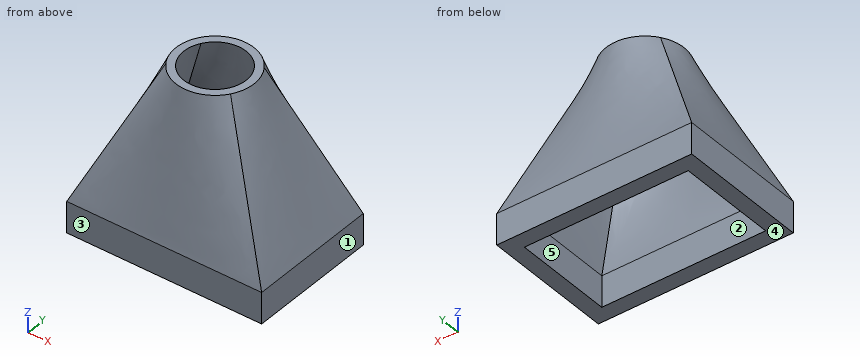
```python
from build123d import *

# Parameters (mm, degrees)
SKETCH1_W           = 12.5
SKETCH1_H           = 8.4
SKETCH1_W_2         = 10.5
SKETCH1_H_2         = 6.4
BOSS_EXTRUDE1_DEPTH = 1
SKETCH6_W           = 12.5
SKETCH6_H           = 8.4
BOSS_EXTRUDE2_DEPTH = 1
SKETCH7_W           = 10.5
SKETCH7_H           = 6.4
CUT_EXTRUDE1_DEPTH  = 1


with BuildPart() as part:
    # Sketch1 → Boss-Extrude1 (new body)
    with BuildSketch(Plane.XY):
        Rectangle(SKETCH1_W, SKETCH1_H)
        Rectangle(SKETCH1_W_2, SKETCH1_H_2, mode=Mode.SUBTRACT)
    extrude(amount=BOSS_EXTRUDE1_DEPTH)

    # Sketch3 → Loft1 section 0
    with BuildSketch(Plane.XY.offset(1)):
        with BuildLine():
            Line((6.25, -4.2), (6.25, 4.2))
            Line((6.25, 4.2), (-6.25, 4.2))
            Line((-6.25, 4.2), (-6.25, -4.2))
            Line((-6.25, -4.2), (6.25, -4.2))
        make_face()
    # Sketch2 for Loft1 → Loft1 section 1
    with BuildSketch(Plane.XY.offset(10)):
        with BuildLine():
            # circular arc as an exact rational Bezier (weights 1, cos(half-angle), 1)
            Bezier((2.075003924, -1.394402637), (3.012042497, 0), (2.075003924, 1.394402637), weights=[1, 0.830001569, 1])
            Bezier((2.075003924, 1.394402637), (0, 4.482206096), (-2.075003924, 1.394402637), weights=[1, 0.557761055, 1])
            Bezier((-2.075003924, 1.394402637), (-3.012042497, 0), (-2.075003924, -1.394402637), weights=[1, 0.830001569, 1])
            Bezier((-2.075003924, -1.394402637), (0, -4.482206096), (2.075003924, -1.394402637), weights=[1, 0.557761055, 1])
        make_face()
    loft()

    # Cut-Loft1: read off the stored shape, not the designer's step
    # Cut-Loft1: loft between two sections, ruled curve by curve
    cut_loft1_from = [
        Edge.make_bspline([(1.707768655, -1.040925656, 10), (1.633699479, -1.162445397, 10), (1.542008876, -1.28354475, 10), (1.31984949, -1.511051231, 10), (1.189256111, -1.617336715, 10), (0.892947872, -1.797985608, 10), (0.72722112, -1.87212471, 10), (0.374256765, -1.973229171, 10), (0.187198335, -2, 10), (-0.187198335, -2, 10), (-0.374256765, -1.973229171, 10), (-0.72722112, -1.87212471, 10), (-0.892947872, -1.797985608, 10), (-1.189256111, -1.617336715, 10), (-1.31984949, -1.511051231, 10), (-1.542008876, -1.28354475, 10), (-1.633699479, -1.162445397, 10), (-1.707768655, -1.040925656, 10)], [0, 0, 0, 0, 0.125, 0.125, 0.25, 0.25, 0.375, 0.375, 0.5, 0.5, 0.625, 0.625, 0.75, 0.75, 0.875, 0.875, 1, 1, 1, 1], 3),
        Edge.make_bspline([(-1.707768655, -1.040925656, 10), (-1.798062507, -0.892787306, 10), (-1.872174068, -0.727085204, 10), (-1.973239973, -0.374182636, 10), (-2, -0.187161202, 10), (-2, 0.187161202, 10), (-1.973239973, 0.374182636, 10), (-1.872174068, 0.727085204, 10), (-1.798062507, 0.892787306, 10), (-1.707768655, 1.040925656, 10)], [0, 0, 0, 0, 0.25, 0.25, 0.5, 0.5, 0.75, 0.75, 1, 1, 1, 1], 3),
        Edge.make_bspline([(1.707768655, 1.040925656, 10), (1.798062507, 0.892787306, 10), (1.872174068, 0.727085204, 10), (1.973239973, 0.374182636, 10), (2, 0.187161202, 10), (2, -0.187161202, 10), (1.973239973, -0.374182636, 10), (1.872174068, -0.727085204, 10), (1.798062507, -0.892787306, 10), (1.707768655, -1.040925656, 10)], [0, 0, 0, 0, 0.25, 0.25, 0.5, 0.5, 0.75, 0.75, 1, 1, 1, 1], 3),
        Edge.make_bspline([(-1.707768655, 1.040925656, 10), (-1.633699479, 1.162445397, 10), (-1.542008876, 1.28354475, 10), (-1.31984949, 1.511051231, 10), (-1.189256111, 1.617336715, 10), (-0.892947872, 1.797985608, 10), (-0.72722112, 1.87212471, 10), (-0.374256765, 1.973229171, 10), (-0.187198335, 2, 10), (0.187198335, 2, 10), (0.374256765, 1.973229171, 10), (0.72722112, 1.87212471, 10), (0.892947872, 1.797985608, 10), (1.189256111, 1.617336715, 10), (1.31984949, 1.511051231, 10), (1.542008876, 1.28354475, 10), (1.633699479, 1.162445397, 10), (1.707768655, 1.040925656, 10)], [0, 0, 0, 0, 0.125, 0.125, 0.25, 0.25, 0.375, 0.375, 0.5, 0.5, 0.625, 0.625, 0.75, 0.75, 0.875, 0.875, 1, 1, 1, 1], 3),
    ]
    cut_loft1_to = [
        Edge.make_bspline([(5.25, -3.2, 1), (4.8125, -3.2, 1), (4.375, -3.2, 1), (3.5, -3.2, 1), (3.0625, -3.2, 1), (2.1875, -3.2, 1), (1.75, -3.2, 1), (0.875, -3.2, 1), (0.4375, -3.2, 1), (-0.4375, -3.2, 1), (-0.875, -3.2, 1), (-1.75, -3.2, 1), (-2.1875, -3.2, 1), (-3.0625, -3.2, 1), (-3.5, -3.2, 1), (-4.375, -3.2, 1), (-4.8125, -3.2, 1), (-5.25, -3.2, 1)], [0, 0, 0, 0, 0.125, 0.125, 0.25, 0.25, 0.375, 0.375, 0.5, 0.5, 0.625, 0.625, 0.75, 0.75, 0.875, 0.875, 1, 1, 1, 1], 3),
        Edge.make_bspline([(-5.25, -3.2, 1), (-5.25, -2.666666667, 1), (-5.25, -2.133333333, 1), (-5.25, -1.066666667, 1), (-5.25, -0.533333333, 1), (-5.25, 0.533333333, 1), (-5.25, 1.066666667, 1), (-5.25, 2.133333333, 1), (-5.25, 2.666666667, 1), (-5.25, 3.2, 1)], [0, 0, 0, 0, 0.25, 0.25, 0.5, 0.5, 0.75, 0.75, 1, 1, 1, 1], 3),
        Edge.make_bspline([(5.25, 3.2, 1), (5.25, 2.666666667, 1), (5.25, 2.133333333, 1), (5.25, 1.066666667, 1), (5.25, 0.533333333, 1), (5.25, -0.533333333, 1), (5.25, -1.066666667, 1), (5.25, -2.133333333, 1), (5.25, -2.666666667, 1), (5.25, -3.2, 1)], [0, 0, 0, 0, 0.25, 0.25, 0.5, 0.5, 0.75, 0.75, 1, 1, 1, 1], 3),
        Edge.make_bspline([(-5.25, 3.2, 1), (-4.8125, 3.2, 1), (-4.375, 3.2, 1), (-3.5, 3.2, 1), (-3.0625, 3.2, 1), (-2.1875, 3.2, 1), (-1.75, 3.2, 1), (-0.875, 3.2, 1), (-0.4375, 3.2, 1), (0.4375, 3.2, 1), (0.875, 3.2, 1), (1.75, 3.2, 1), (2.1875, 3.2, 1), (3.0625, 3.2, 1), (3.5, 3.2, 1), (4.375, 3.2, 1), (4.8125, 3.2, 1), (5.25, 3.2, 1)], [0, 0, 0, 0, 0.125, 0.125, 0.25, 0.25, 0.375, 0.375, 0.5, 0.5, 0.625, 0.625, 0.75, 0.75, 0.875, 0.875, 1, 1, 1, 1], 3),
    ]
    cut_loft1 = Solid(Shell([*[Face.make_surface_from_curves(cut_loft1_from[k], cut_loft1_to[k]) for k in range(4)], Face(Wire(cut_loft1_from)), Face(Wire(cut_loft1_to))]))
    add(cut_loft1, mode=Mode.SUBTRACT)

    # Sketch6 → Boss-Extrude2 (add)
    with BuildSketch(Plane(origin=(0, 0, 0), x_dir=(-1, 0, 0), z_dir=(0, 0, -1))):
        Rectangle(SKETCH6_W, SKETCH6_H)
    extrude(amount=BOSS_EXTRUDE2_DEPTH)

    # Sketch7 → Cut-Extrude1 (cut)
    with BuildSketch(Plane(origin=(0, 0, -1), x_dir=(-1, 0, 0), z_dir=(0, 0, -1))):
        Rectangle(SKETCH7_W, SKETCH7_H)
    extrude(amount=-CUT_EXTRUDE1_DEPTH, mode=Mode.SUBTRACT)


solid = part.part
```
The listing builds one solid part. Answer for the finished solid, in the listing's coordinates (mm). Face numbers are marked on the shaded views. A direction names the side the tool comes from. Round coordinates to 2 decimals unless told otherwise and drop trailing zeros.
Q1. Given pin 1 Ø5 at (x, z) = (3, 5) entering from -Y; pin 2 Ø3 at (x, y) = (-1, -2) entering from -Z; pin 3 Ø4 at (y, z) = (-0.5, 5) entering from -X, each flat-ended and moving along its own axis, determine where each tip first touches the part or whether it passes through.
Q2. For a pull along Y with two mould halves and no side action, classify the marked faces 1, 2 and 3 as released by +Y, released by -Y, zero draft, split by the parting line, or undercut.
Q3. Find the intervals of material crossed by line 1 (X direction, y = -0.75, z = 1); line 2 (Y direction, x = 4, z = 0.5); line 3 (X direction, y = -0.75, z = 6.75), in increasing order.
Q4. Which of the six approach directions +Z, -Z, +X, -X, +Y, -Y give full straight-line access (tool end or side, diameter ignored) to the marked faces 4 and 5?
Completed:
1. pin 1: stops at y = -3.86
1. pin 2: stops at z = -1
1. pin 3: stops at x = -5.41
2. face 1: zero draft
2. face 2: undercut
2. face 3: released by -Y
3. line 1: x = -6.25 to -5.25, 5.25 to 6.25
3. line 2: y = -4.2 to -3.2, 3.2 to 4.2
3. line 3: x = -3.83 to -3.14, 3.14 to 3.83
4. face 4: -Z, +X, -X, +Y, -Y
4. face 5: -Z
